from build123d import *

# Parameters (mm, degrees)
SKETCH1_W           = 26.25
SKETCH1_H           = 15
SKETCH1_R           = 1.5
BOSS_EXTRUDE1_DEPTH = 1


with BuildPart() as part:
    # Sketch1 → Boss-Extrude1 (new body, symmetric)
    with BuildSketch(Plane(origin=(0, 0, 0), x_dir=(1, 0, 0), z_dir=(0, 1, 0))):
        Rectangle(SKETCH1_W, SKETCH1_H)
        with Locations((-10.625, 5.5)):
            Circle(SKETCH1_R, mode=Mode.SUBTRACT)
        with Locations((10.625, 5.5)):
            Circle(SKETCH1_R, mode=Mode.SUBTRACT)
    extrude(amount=BOSS_EXTRUDE1_DEPTH, both=True)


solid = part.part
The listing builds one solid part. Answer for the finished solid, in the listing's coordinates (mm). Coordinates: 2 decimals unless noted, no trailing zeros. Order: outer loops, then holes, each group sorted by start corner. A loop starts at its lowest first (then second) coordinate and runs counter-clockwise, first axis right, second up. Notation, with made-up numbers: (58, -38.75) -> (110, -38.75) arc R20 ccw to (110, -31.75) -> close; hole circle Ø4 at (-20, 37.25). An arc over 180 degrees is marked (long way). Answer in a Markdown table with one row per item. Add a question column.
Item 1: Determine the mould class of faces 1 (the face through (0, 0, -7.5)), 2 (the face through (-12.124, -0.014, -5.566)), 3 (the face through (9.126, -0.014, -5.566)), 4 (the face through (0, 1, 0)) for opening direction Z: +Z half, -Z half, draft (parallel to the pull), parting line (faces both ways), or undercut.
Item 2: Find section A-A (z = -5.5). Write down the section's boundary in (x, y) (3 decimals).
Item 3: Find the intervals of material crossed by L1, parallel to X at y = 0.05, z = -5.5 (3 decimals); L2, parallel to X at y = -0.1, z = -6.75 (3 decimals); L3, parallel to Z at x = -11, y = 0.2, in increasing order. Write a range as from..to.
Item 4: Find section B-B (x = -11). Write down the section's boundary in (y, z).
Item 5: Find section C-C (y = 0.25). Write down the section's boundary in (x, z) (3 decimals), then the cut area to 3 significant figures.
Result set:
| question | item | result |
|---|---|---|
| 1 | face 1 | -Z half |
| 1 | face 2 | undercut |
| 1 | face 3 | undercut |
| 1 | face 4 | draft |
| 2 | outline | (-13.125, -1) -> (-12.125, -1) -> (-12.125, 1) -> (-13.125, 1) -> close; (-9.125, -1) -> (9.125, -1) -> (9.125, 1) -> (-9.125, 1) -> close; (12.125, -1) -> (13.125, -1) -> (13.125, 1) -> (12.125, 1) -> close |
| 3 | L1 | x = -13.125..-12.125, -9.125..9.125, 12.125..13.125 |
| 3 | L2 | x = -13.125..-11.454, -9.796..9.796, 11.454..13.125 |
| 3 | L3 | z = -7.5..-6.95, -4.05..7.5 |
| 4 | outline | (-1, -7.5) -> (1, -7.5) -> (1, -6.95) -> (-1, -6.95) -> close; (-1, -4.05) -> (1, -4.05) -> (1, 7.5) -> (-1, 7.5) -> close |
| 5 | outline | (-13.125, -7.5) -> (13.125, -7.5) -> (13.125, 7.5) -> (-13.125, 7.5) -> close; hole circle Ø3 at (-10.625, -5.5); hole circle Ø3 at (10.625, -5.5) |
| 5 | area | 380 mm² |
